from build123d import *

# Parameters (mm, degrees)
SKETCH_1_R          = 4
EXTRUDE_1_DEPTH     = 6.5
SKETCH_2_R          = 3.5
EXTRUDE_2_DEPTH     = 8.5
SKETCH_3_R          = 1.5
CUT_EXTRUDE_1_DEPTH = 107.248752968


with BuildPart() as part:
    # 草图1 → 凸台-拉伸1 (new body)
    with BuildSketch(Plane(origin=(0, 0, 0), x_dir=(1, 0, 0), z_dir=(0, 1, 0))):
        with BuildLine():
            ThreePointArc((0, 5), (-4.999517366, -0.06947017), (0.138926929, -4.998069558))
            Line((0.138926929, -4.998069558), (99.990347325, -3.61059659))
            ThreePointArc((99.990347325, -3.61059659), (104.990347325, 1.38940341), (99.990347325, 6.38940341))
            Line((99.990347325, 6.38940341), (0, 5))
        make_face()
        with Locations(Location((0, 0, 0), (0, 0, 90))):
            Circle(SKETCH_1_R, mode=Mode.SUBTRACT)
    extrude(amount=EXTRUDE_1_DEPTH)

    # 草图2 → 凸台-拉伸2 (add)
    with BuildSketch(Plane(origin=(0, 6.5, 0), x_dir=(1, 0, 0), z_dir=(0, 1, 0))):
        with Locations(Location((99.990347325, 1.38940341, 0), (0, 0, 270))):
            Circle(SKETCH_2_R)
    extrude(amount=EXTRUDE_2_DEPTH)

    # 草图3 → 切除-拉伸1 (cut, through all)
    with BuildSketch(Plane(origin=(0, 15, 0), x_dir=(1, 0, 0), z_dir=(0, 1, 0))):
        with Locations(Location((99.990347325, 1.38940341, 0), (0, 0, 270))):
            Circle(SKETCH_3_R)
    extrude(amount=-CUT_EXTRUDE_1_DEPTH, mode=Mode.SUBTRACT)


solid = part.part
Input: part model. Units: mm. Frame: model coordinates. Coordinates: 2 decimals unless noted, no trailing zeros. Loops run counter-clockwise (first coordinate to the right, second up) from the corner with the lowest first, then second, coordinate; pieces in that order, holes last. Notation, with made-up numbers: (38, 62.25) -> (84, 62.25) arc R16 ccw to (84, 86.25) -> close; hole circle Ø10 at (-29.75, 2). An arc over 180 degrees is marked (long way). One line per item, written item: value.
(1) Draft query along Z for faces 1 (the face through (103.46, 10.69, -1.85)), 2 (the face through (98.66, 7.6, -0.7)), 3 (the face through (49, 0, -1)). Return one class per face: pulls with the +Z half, pulls with the -Z half, needs draft (parallel to the pull), parting line crosses it, or undercut.
Answer below:
face 1: parting line crosses it
face 2: undercut
face 3: needs draft
(2) Pin query (flat end, axial travel): pin 1 Ø4 at (x, z) = (37, 1) entering from -Y; pin 2 Ø2 at (y, z) = (4, -3.5) entering from +X; pin 3 Ø1.5 at (y, z) = (5.5, -4) entering from -X; pin 4 Ø1.8 at (x, z) = (99.99, -1.39) entering from -Y. Return the tip coordinate at first contact, or that it passes through.
Answer below:
pin 1: stops at y = 0
pin 2: stops at x = 104.87
pin 3: stops at x = -3.8
pin 4: passes through
(3) Cut plane A-A (y = 11). Output: boundary loops of the cut face in (x, z).
Answer below:
outline: circle Ø7 at (99.99, -1.39); hole circle Ø3 at (99.99, -1.39)
(4) Ray query, line 1 along X through (y, z) = (5.5, -1.75); line 2 along Y through (x, z) = (11.5, 4.5); line 3 along X through (y, z) = (2, -1). Return the intervals inside material, ascending.
Answer below:
line 1: x = -4.68 to -3.6, 3.6 to 98.53, 101.45 to 104.98
line 2: y = 0 to 6.5
line 3: x = -4.9 to -3.87, 3.87 to 98.54, 101.44 to 104.98
(5) Cut plane B-B (x = 74). Output: boundary loops of the cut face in (y, z), then the cut area to 3 significant figures.
Answer below:
outline: (0, -6.03) -> (6.5, -6.03) -> (6.5, 3.97) -> (0, 3.97) -> close
area: 65.0 mm2
